```python
from build123d import *

# Parameters (mm, degrees)
F0_W        = 152.4
F0_H        = 304.8
F1_DEPTH    = 25.4
F2_T1_DEPTH = 1081.4461668656
F3_W        = 57.15
F3_H        = 57.15
F4_DEPTH    = 25.4


# Not quite as in the source:
# - a fillet or chamfer that OpenCascade refuses, or shapes differently, is made with other operations: its cross-section is extruded or revolved along the edge and cut away or added


with BuildPart() as f1:
    # F0 (on Front) → F1 (new body)
    with BuildSketch(Plane.XZ):
        with Locations((-29.3548897063, -4.3910965323)):
            Rectangle(F0_W, F0_H)
    extrude(amount=F1_DEPTH)

    # F2: chamfer of 203.2 x 35.82964248 on 1 edges, made by hand

    # F2_s2 → F2_t1 (cut)
    with BuildSketch(Plane.XZ.offset(-528.0230834328)):
        Polygon((97.6451102937, 148.0089034677), (-105.5548897063, 112.1792609877), (-105.5548897063, 148.0089034677), align=None)
    extrude(amount=F2_T1_DEPTH, mode=Mode.SUBTRACT)

    # F3 (on face) → F4 (cut, through all)
    with BuildSketch(Plane.XZ):
        with Locations((-28.575, 59.6764928477)):
            Rectangle(F3_W, F3_H)
    extrude(amount=F4_DEPTH, mode=Mode.SUBTRACT)


solid = f1.part
```
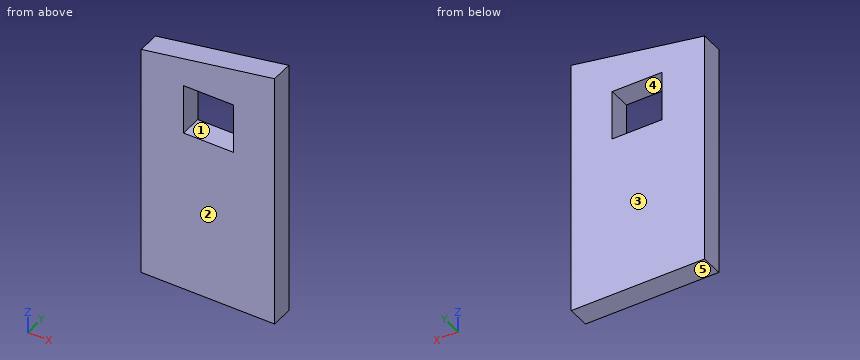
Part model, mm, in its own coordinate system. Face numbers are marked on the shaded views. A direction names the side the tool comes from. Give positions to 0.01 mm unless a question says otherwise; leave off trailing zeros. Write each loop counter-clockwise with the first axis right and the second up, starting at its lowest first coordinate (ties: lowest second). Pieces come first, ordered by that corner, then holes. Notation, with made-up numbers: (66, 33.25) -> (98, 33.25) arc R32 ccw to (98, 63.25) -> close; hole circle Ø8 at (4, -5). An arc over 180 degrees is marked (long way). Put each result on its own line as item: value. Start each with the question number.
Item 1: Cut at D-D (x = 12). List the corners of the cut face in (y, z).
Item 2: Cut at A-A (z = 75.5). List the corners of the cut face in (x, y), then the cut area to 3 significant figures.
Item 3: Which spindle directions (+Z, -Z, +X, -X, +Y, -Y) get a long thin tool onto all of the face, cutting with end or side? Do the marked faces 1 and 2. Say none if no direction does.
Item 4: Cut at B-B (y = -10). List the corners of the cut face in (x, z), then the cut area to 3 significant figures.
Item 5: Wall check: L1, parallel to X at y = -15.25, z = 76.5; L2, parallel to Z at x = -3, y = -19; L3, parallel to Z at x = -66, y = -8. Give the ranges that are in metal, low to high. Write a range as [from, to].
Item 6: Cut at C-C (x = -79). List the corners of the cut face in (y, z).
Item 7: Pull direction Z, two halves, no side cores. Call the marked faces 3, 4 and 5: pulls with the +Z half, pulls with the -Z half, needs draft (parallel to the pull), parting line crosses it, or undercut.
Answer list:
1. outline: (-25.4, -156.79) -> (0, -156.79) -> (0, 132.91) -> (-25.4, 132.91) -> close
2. outline: (-105.55, -25.4) -> (-57.15, -25.4) -> (-57.15, 0) -> (-105.55, 0) -> close; (0, -25.4) -> (46.85, -25.4) -> (46.85, 0) -> (0, 0) -> close
2. area: 2,420 mm2
3. face 1: +Y, -Y
3. face 2: +Z, -Z, +X, -X, -Y
4. outline: (-105.55, -156.79) -> (46.85, -156.79) -> (46.85, 139.05) -> (-105.55, 112.18) -> close; hole (-57.15, 31.1) -> (0, 31.1) -> (0, 88.25) -> (-57.15, 88.25) -> close
4. area: 39,800 mm2
5. L1: x = [-105.55, -57.15], [0, 46.85]
5. L2: z = [-156.79, 31.1], [88.25, 130.26]
5. L3: z = [-156.79, 119.15]
6. outline: (-25.4, -156.79) -> (0, -156.79) -> (0, 116.86) -> (-25.4, 116.86) -> close
7. face 3: needs draft
7. face 4: undercut
7. face 5: pulls with the -Z half
